Design review of the part shown in the three views and the two pictorial views. Dimensions are in mm from the part's minimum x, y and z. A direction names the side the tool comes from. Coordinates: 2 decimals unless noted, no trailing zeros. One line per item, written item: value.
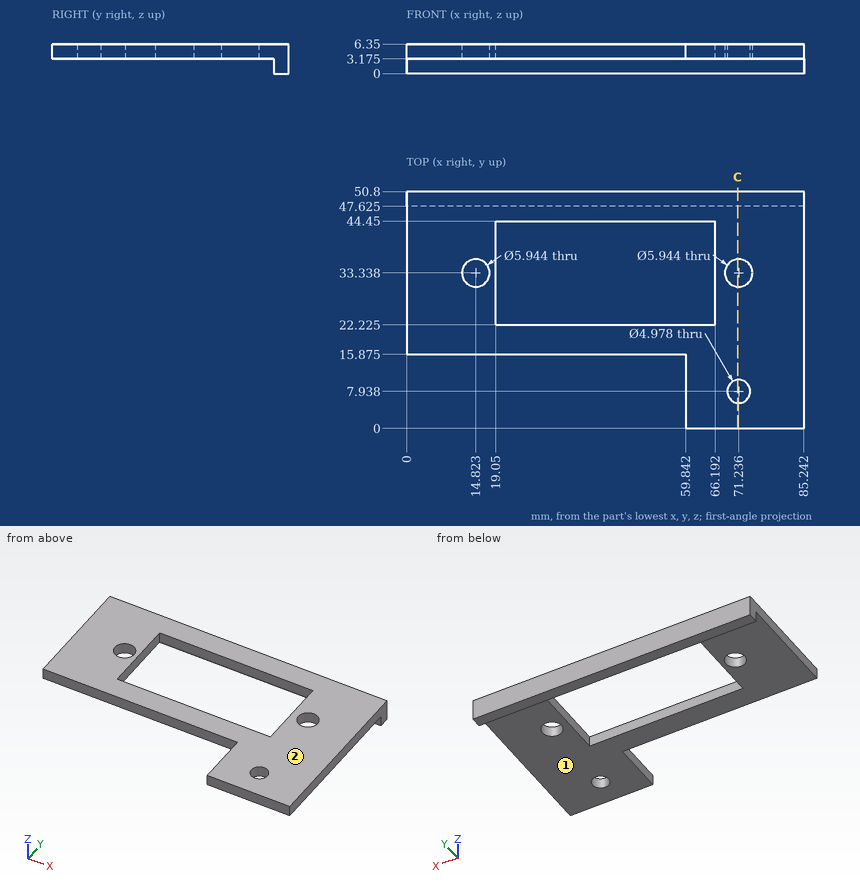
1. Take a section at C-C, the plane x = 71. Give the number of separate pieces and of enclosed holes in the cut face, and give its area (3 significant figures).
Return value:
separate pieces: 3
enclosed holes: 0
area: 137 mm2
2. To check wall thickness, follow probe 1 along X at (y, z) = (27.5, 4.5); probe 2 along Y at (x, z) = (22.5, 2) (1 decimal); probe 3 along Y at (x, z) = (69, 5.5) (1 decimal). State the ranges of each line that lie inside material, in increasing order. Write a range as from..to.
Return value:
probe 1: x = 0..19.05, 66.19..85.24
probe 2: y = 47.6..50.8
probe 3: y = 0..6.8, 9..31.4, 35.3..50.8
3. For the marked faces 1 and 2, list the 3-axis set-ups (+Z, -Z, +X, -X, +Y, -Y) from which the entire face can be reached by the end or side of a thin tool; tool diameter is ignored.
Return value:
face 1: -Z, +X, -X, -Y
face 2: +Z, +X, -X, +Y, -Y
4. Insertion check: pin 1 Ø14.5 at (x, y) = (49.5, 18) entering from -Z (1 decimal); pin 2 Ø1.6 at (x, z) = (34.5, 5) entering from -Y (1 decimal); pin 3 Ø1.6 at (x, z) = (44.5, 1.5) entering from -Y (1 decimal). Each pin has a flat end and moves straight along its axis. Give the tip position at first contact, or say it passes through.
Return value:
pin 1: stops at z = 3.2
pin 2: stops at y = 15.9
pin 3: stops at y = 47.6
